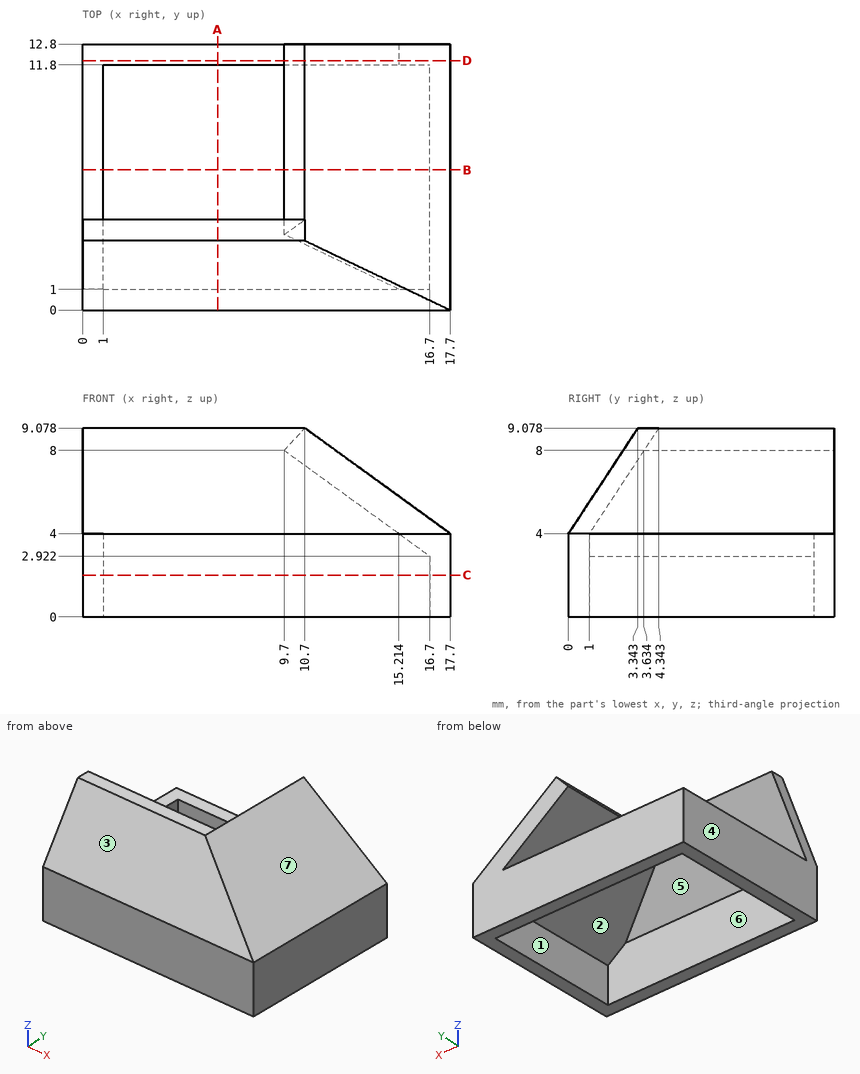
Job drawing, mm, ordinate dimensions from the low corner. One solid piece. A direction names the side the tool comes from. Give positions to 0.01 mm unless a question says otherwise; leave off trailing zeros. Order: outer loops, then holes, each group sorted by start corner. A loop starts at its lowest first (then second) coordinate and runs counter-clockwise, first axis right, second up. Notation, with made-up numbers: (77.5, 18) - (132.5, 18) arc R21 ccw to (132.5, 36) - close; hole circle Ø4 at (54, -8.75). An arc over 180 degrees is marked (long way). Return JSON: item names as keys, results as strings.
1) Cut at C-C, the plane z = 2. Give the cut face in (x, y).
Geometry says:
{"outline": "(0, 0) - (17.7, 0) - (17.7, 12.8) - (0, 12.8) - close; hole (1, 1) - (16.7, 1) - (16.7, 11.8) - (1, 11.8) - close"}
2) Flat gauge pins, fed straight in: P1, Ø1.5, axis at y = 10.5, z = 5, coming from the +X side (1 decimal); P2, Ø1.5, axis at x = 8, y = 9.5, coming from the -Z side. Where does each tip first touch, or does it go through?
Geometry says:
{"P1": "x = 17.4", "P2": "through"}
3) Pull direction Y, two halves, no side cores. Call the marked faces 1, 2, 3 and 4: pulls with the +Y half, pulls with the -Y half, needs draft (parallel to the pull), parting line crosses it, or undercut.
Geometry says:
{"face 1": "undercut", "face 2": "undercut", "face 3": "pulls with the -Y half", "face 4": "needs draft"}
4) 3-axis set-ups, long thin cutter, end or side, ignore diameter. For the marked faces 5, 6 and 7: which of +Z, -Z, +X, -X, +Y, -Y reach the whole face in a straight line?
Geometry says:
{"face 5": "-X, +Y", "face 6": "-Z", "face 7": "+Z, +X, +Y, -Y"}
5) Cut at D-D, the plane y = 12. Give the cut face in (x, z) (1 decimal).
Geometry says:
{"outline": "(0, 0) - (17.7, 0) - (17.7, 4) - (10.7, 9.1) - (9.7, 8) - (15.2, 4) - (0, 4) - close"}
6) Cut at A-A, the plane x = 6.5. Give the cut face in (y, z).
Geometry says:
{"outline": "(0, 0) - (1, 0) - (1, 4) - (4.34, 9.08) - (3.34, 9.08) - (0, 4) - close; (11.8, 0) - (12.8, 0) - (12.8, 4) - (11.8, 4) - close"}
7) Probe line 1 (Y direction, x = 13.25, z = 2.5); line 2 (X direction, y = 10.75, z = 3.75); line 3 (X direction, y = 4.5, z = 4.25) (1 decimal). List the from-to ranges inside material, lowest first. Write a range as from..to.
Geometry says:
{"line 1": "0..1, 11.8..12.8", "line 2": "0..1, 15.56..17.7", "line 3": "14.9..17.4"}
8) Cut at B-B, the plane y = 6.75. Give the cut face in (x, z).
Geometry says:
{"outline": "(0, 0) - (1, 0) - (1, 4) - (0, 4) - close; (9.7, 8) - (16.7, 2.92) - (16.7, 0) - (17.7, 0) - (17.7, 4) - (10.7, 9.08) - close"}
